Work out the finished part from the listing and answer in its coordinate system (mm). A direction names the side the tool comes from. Coordinates: 2 decimals unless noted, no trailing zeros. Order: outer loops, then holes, each group sorted by start corner. A loop starts at its lowest first (then second) coordinate and runs counter-clockwise, first axis right, second up. Notation, with made-up numbers: M 82.5,3.5 L 114.5,3.5 A11 cw 114.5,14.5 Z; hole C 77,56.25 d10. An arc over 180 degrees is marked long. Use a Markdown table: item, result.
from build123d import *

# Parameters (mm, degrees)
F1_DEPTH = 25.4


# Not quite as in the source:
# - a feature names something its author has since deleted; it is built from what else it names


with BuildPart() as f1:
    # F0 (on Front) → F1 (new body)
    with BuildSketch(Plane.XZ):
        with BuildLine():
            Line((-1.9275679621, -0.9906), (2.0602320379, -0.9906))
            Line((2.0602320379, -0.9906), (2.0602320379, 2.9972))
            ThreePointArc((2.0602320379, 2.9972), (1.7808320379, 3.1758966119), (1.5014320379, 2.9972))
            Line((1.5014320379, 2.9972), (0.2927852911, 0.381))
            Line((0.2927852911, 0.381), (-0.2070155831, 0.3918310395))
            Line((-0.2070155831, 0.3918310395), (-1.3567524399, 2.9972))
            ThreePointArc((-1.3567524399, 2.9972), (-1.642160201, 3.1832136759), (-1.9275679621, 2.9972))
            Line((-1.9275679621, 2.9972), (-1.9275679621, -0.9906))
        make_face()
        with BuildLine():
            ThreePointArc((1.5014320379, 2.9972), (1.7808320379, 3.1758966119), (2.0602320379, 2.9972))
            Line((2.0602320379, 2.9972), (2.0602320379, 4.8607838479))
            Line((2.0602320379, 4.8607838479), (0.575090351, 4.8607838479))
            Line((0.575090351, 4.8607838479), (0.575090351, 4.3721500923))
            Line((0.575090351, 4.3721500923), (1.5014320379, 4.3721500923))
            Line((1.5014320379, 4.3721500923), (1.5014320379, 2.9972))
        make_face()
    extrude(amount=F1_DEPTH)


solid = f1.part
1. Find the intervals of material crossed by probe 1 along X at (y, z) = (-2, 4.6); probe 2 along X at (y, z) = (-22, 0.9); probe 3 along Z at (x, y) = (1.15, -15.75), in increasing order.
Answers below:
| item | result |
|---|---|
| probe 1 | 0.58 to 2.06 |
| probe 2 | -1.93 to -0.43, 0.53 to 2.06 |
| probe 3 | -0.99 to 2.24, 4.37 to 4.86 |
2. For a pull along Z with two mould halves and no side action, classify faces 1 (the face through (-1.928, -13, 1)), 2 (the face through (1, -13, 4.372)), 3 (the face through (-0.774, -12.522, 1.676)) as +Z half, -Z half, draft (parallel to the pull), parting line (faces both ways), or undercut.
Answers below:
| item | result |
|---|---|
| face 1 | draft |
| face 2 | undercut |
| face 3 | +Z half |
3. Section D-D on x = -0.45 is taken. Determine the outline of the cut face in (y, z).
Answers below:
| item | result |
|---|---|
| outline | M -25.4,-0.99 L 0,-0.99 L 0,0.94 L -25.4,0.94 Z |
4. Section C-C on x = 1.2 is taken. Determine the outline of the cut face in (y, z).
Answers below:
| item | result |
|---|---|
| outline | M -25.4,-0.99 L 0,-0.99 L 0,2.34 L -25.4,2.34 Z; M -25.4,4.37 L 0,4.37 L 0,4.86 L -25.4,4.86 Z |
5. Section B-B on y = -12 is taken. Determine the outline of the cut face in (x, z).
Answers below:
| item | result |
|---|---|
| outline | M -1.93,-0.99 L 2.06,-0.99 L 2.06,4.86 L 0.58,4.86 L 0.58,4.37 L 1.5,4.37 L 1.5,3 L 0.29,0.38 L -0.21,0.39 L -1.36,3 A0.31 ccw -1.93,3 Z |
6. For faces 4 (the face through (1, -25.4, 1)), 5 (the face through (0.9, -12.5, 1.7)), determine the directions among +Z, -Z, +X, -X, +Y, -Y from which every point of the face is accessible in a straight line to the end or side of a thin tool.
Answers below:
| item | result |
|---|---|
| face 4 | +Z, -Z, +X, -X, -Y |
| face 5 | +Y, -Y |
7. Section A-A on z = 1.25 is taken. Determine the outline of the cut face in (x, y).
Answers below:
| item | result |
|---|---|
| outline | M -1.93,-25.4 L -0.59,-25.4 L -0.59,0 L -1.93,0 Z; M 0.69,-25.4 L 2.06,-25.4 L 2.06,0 L 0.69,0 Z |
